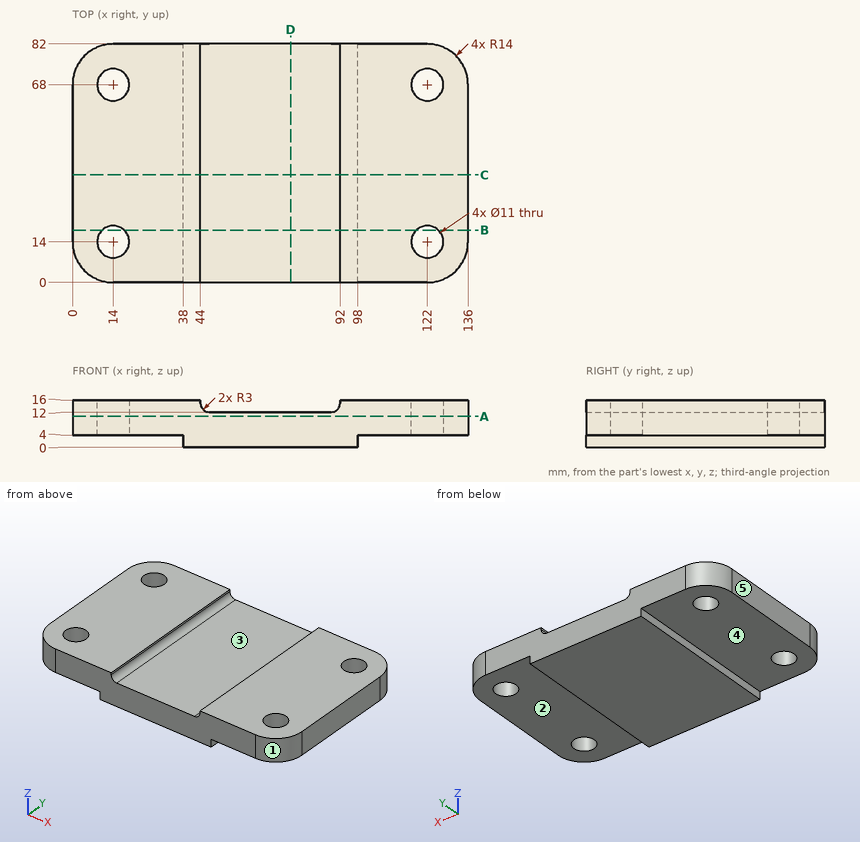
The figure shows three views and two pictorial views of one solid part (mm, origin at its lowest corner). Answer the questions. A direction names the side the tool comes from. Round coordinates to 2 decimals unless told otherwise and drop trailing zeros. Write each loop counter-clockwise with the first axis right and the second up, starting at its lowest first coordinate (ties: lowest second). Pieces come first, ordered by that corner, then holes. Notation, with made-up numbers: (-21, 1.5) -> (-6, 1.5) arc R17 cw to (-6, 9.5) -> close; hole circle Ø2 at (41.5, 20.5). An arc over 180 degrees is marked (long way). Write each question's results on one line, items separated by ' | '.
Q1. Determine the mould class of the marked faces 1, 2 and 3 for opening direction X: released by +X, released by -X, zero draft, split by the parting line, or undercut.
Data:
face 1: released by +X | face 2: zero draft | face 3: undercut
Q2. Section A-A, the plane z = 10.5 is taken. Write down the section's boundary in (x, y).
Data:
outline: (0, 14) arc R14 ccw to (14, 0) -> (122, 0) arc R14 ccw to (136, 14) -> (136, 68) arc R14 ccw to (122, 82) -> (14, 82) arc R14 ccw to (0, 68) -> close; hole circle Ø11 at (14, 14); hole circle Ø11 at (14, 68); hole circle Ø11 at (122, 14); hole circle Ø11 at (122, 68)
Q3. Flat-ended cylindrical pins translate along their axes: P1, Ø11.5, axis at x = 115, y = 33, coming from the -Z side; P2, Ø6, axis at y = 10.5, z = 9.5, coming from the +X side; P3, Ø1, axis at x = 69.5, z = 13, coming from the -Y side; P4, Ø3, axis at x = 76, y = 27.5, coming from the +Z side. Find the tip coordinate at first contact, or state that the pin passes through.
Data:
P1: z = 4 | P2: x = 135.99 | P3: through | P4: z = 12
Q4. Section D-D, the plane x = 75 is taken. Write down the section's boundary in (y, z), then the cut area to 3 significant figures.
Data:
outline: (0, 0) -> (82, 0) -> (82, 12) -> (0, 12) -> close | area: 984 mm^2
Q5. Straight lines are drawn through the part: line 1 along Y through (x, z) = (122, 9.75); line 2 along X through (y, z) = (67.5, 6.25); line 3 along X through (y, z) = (39, 3). For each, find the intervals that lie inside material, in ascending order. Write a range as [from, to].
Data:
line 1: [0, 8.5], [19.5, 62.5], [73.5, 82] | line 2: [0, 8.52], [19.48, 116.52], [127.48, 136] | line 3: [38, 98]
Q6. Which of the six approach directions +Z, -Z, +X, -X, +Y, -Y give full straight-line access (tool end or side, diameter ignored) to the marked faces 4 and 5?
Data:
face 4: -Z, -X, +Y, -Y | face 5: +Z, -Z, -X, +Y, -Y
Q7. Section C-C, the plane y = 37 is taken. Write down the section's boundary in (x, z), then the cut area to 3 significant figures.
Data:
outline: (0, 4) -> (38, 4) -> (38, 0) -> (98, 0) -> (98, 4) -> (136, 4) -> (136, 16) -> (92, 16) -> (92, 15) arc R3 cw to (89, 12) -> (47, 12) arc R3 cw to (44, 15) -> (44, 16) -> (0, 16) -> close | area: 1,680 mm^2
Q8. Section B-B, the plane y = 18 is taken. Write down the section's boundary in (x, z), then the cut area to 3 significant figures.
Data:
outline: (0, 4) -> (10.23, 4) -> (10.23, 16) -> (0, 16) -> close; (17.77, 4) -> (38, 4) -> (38, 0) -> (98, 0) -> (98, 4) -> (118.23, 4) -> (118.23, 16) -> (92, 16) -> (92, 15) arc R3 cw to (89, 12) -> (47, 12) arc R3 cw to (44, 15) -> (44, 16) -> (17.77, 16) -> close; (125.77, 4) -> (136, 4) -> (136, 16) -> (125.77, 16) -> close | area: 1,500 mm^2
